```python
from build123d import *

# Parameters (mm, degrees)
F0_W      = 90
F0_H      = 19.25
F0_W_2    = 85
F0_H_2    = 12
F1_DEPTH  = 45
F0_W_3    = 7.85
F0_H_3    = 4.66
F2_DEPTH  = 14
F0_R      = 1.5
F3_DEPTH  = 8
F5_W      = 4
F5_H      = 29.0582341515
F6_DEPTH  = 3.07077
F5_H_2    = 15.9417658485
F7_DEPTH  = 8.2825263962
F11_DEPTH = 23.33121
F12_DEPTH = 2.5
F14_W     = 3
F14_H     = 4.4074529409
F14_W_2   = 3.907799057
F14_H_2   = 3
F15_DEPTH = 3


with BuildPart() as f1:
    # F0 (on Front) → F1 (new body)
    with BuildSketch(Plane.XZ):
        with Locations((-17.1932545304, 37.9297346771)):
            Rectangle(F0_W, F0_H)
        with Locations((-17.2074458234, 37.7867133319)):
            Rectangle(F0_W_2, F0_H_2, mode=Mode.SUBTRACT)
    extrude(amount=F1_DEPTH)

    # F0 (on Front) → F2 (join)
    with BuildSketch(Plane.XZ):
        with Locations((-17.2074458234, 37.7867133319)):
            Rectangle(F0_W_2, F0_H_2)
        with Locations((-17.2074458234, 37.7867133319)):
            Rectangle(F0_W_3, F0_H_3, mode=Mode.SUBTRACT)
    extrude(amount=F2_DEPTH)

    # F0 (on Front) → F3 (join)
    with BuildSketch(Plane.XZ):
        with Locations((-17.2074458234, 37.7867133319)):
            Rectangle(F0_W_3, F0_H_3)
        with Locations((-17.2074458234, 37.7867133319)):
            Circle(F0_R, mode=Mode.SUBTRACT)
    extrude(amount=F3_DEPTH)

    # F5 (on offset) → F6 (cut)
    with BuildSketch(Plane(origin=(0, 0, 28.3047346771), x_dir=(1, 0, 0), z_dir=(0, 0, -1))):
        with Locations((-17.1932545304, 30.4708829243)):
            Rectangle(F5_W, F5_H)
    extrude(amount=-F6_DEPTH, mode=Mode.SUBTRACT)

    # F5 (on offset) → F7 (cut)
    with BuildSketch(Plane(origin=(0, 0, 28.3047346771), x_dir=(1, 0, 0), z_dir=(0, 0, -1))):
        with Locations((-17.1932545304, 30.4708829243)):
            Rectangle(F5_W, F5_H)
        with Locations((-17.1932545304, 7.9708829243)):
            Rectangle(F5_W, F5_H_2)
    extrude(amount=-F7_DEPTH, mode=Mode.SUBTRACT)

    # F10 (on offset) → F11 (cut)
    with BuildSketch(Plane(origin=(0, 0, 28.3047346771), x_dir=(1, 0, 0), z_dir=(0, 0, -1))):
        with BuildLine():
            Line((-49.1650958551, 7.0774606429), (-45.4150958551, 7.0774606429))
            ThreePointArc((-45.4150958551, 7.0774606429), (-47.2900958551, 8.9524606429), (-49.1650958551, 7.0774606429))
        make_face()
        with BuildLine():
            ThreePointArc((-49.1650958551, 7.0774606429), (-47.2900958551, 5.2024606429), (-45.4150958551, 7.0774606429))
            Line((-45.4150958551, 7.0774606429), (-49.1650958551, 7.0774606429))
        make_face()
        with BuildLine():
            ThreePointArc((10.8743589147, 7.0774606429), (8.9993589147, 8.9524606429), (7.1243589147, 7.0774606429))
            Line((7.1243589147, 7.0774606429), (10.8743589147, 7.0774606429))
        make_face()
        with BuildLine():
            Line((10.8743589147, 7.0774606429), (7.1243589147, 7.0774606429))
            ThreePointArc((7.1243589147, 7.0774606429), (8.9993589147, 5.2024606429), (10.8743589147, 7.0774606429))
        make_face()
    extrude(amount=-F11_DEPTH, mode=Mode.SUBTRACT)

    # F10 (on offset) → F12 (cut)
    with BuildSketch(Plane(origin=(0, 0, 28.3047346771), x_dir=(1, 0, 0), z_dir=(0, 0, -1))):
        with BuildLine():
            Line((7.1243589147, 7.0774606429), (5.4493589147, 7.0774606429))
            ThreePointArc((5.4493589147, 7.0774606429), (8.9993589147, 3.5274606429), (12.5493589147, 7.0774606429))
            Line((12.5493589147, 7.0774606429), (10.8743589147, 7.0774606429))
            ThreePointArc((10.8743589147, 7.0774606429), (8.9993589147, 5.2024606429), (7.1243589147, 7.0774606429))
        make_face()
        with BuildLine():
            ThreePointArc((12.5493589147, 7.0774606429), (8.9993589147, 10.6274606429), (5.4493589147, 7.0774606429))
            Line((5.4493589147, 7.0774606429), (7.1243589147, 7.0774606429))
            ThreePointArc((7.1243589147, 7.0774606429), (8.9993589147, 8.9524606429), (10.8743589147, 7.0774606429))
            Line((10.8743589147, 7.0774606429), (12.5493589147, 7.0774606429))
        make_face()
        with BuildLine():
            Line((-43.7400958551, 7.0774606429), (-45.4150958551, 7.0774606429))
            ThreePointArc((-45.4150958551, 7.0774606429), (-47.2900958551, 5.2024606429), (-49.1650958551, 7.0774606429))
            Line((-49.1650958551, 7.0774606429), (-50.8400958551, 7.0774606429))
            ThreePointArc((-50.8400958551, 7.0774606429), (-47.2900958551, 3.5274606429), (-43.7400958551, 7.0774606429))
        make_face()
        with BuildLine():
            ThreePointArc((-49.1650958551, 7.0774606429), (-47.2900958551, 8.9524606429), (-45.4150958551, 7.0774606429))
            Line((-45.4150958551, 7.0774606429), (-43.7400958551, 7.0774606429))
            ThreePointArc((-43.7400958551, 7.0774606429), (-47.2900958551, 10.6274606429), (-50.8400958551, 7.0774606429))
            Line((-50.8400958551, 7.0774606429), (-49.1650958551, 7.0774606429))
        make_face()
    extrude(amount=-F12_DEPTH, mode=Mode.SUBTRACT)

    # F14 (on face) → F15 (cut)
    with BuildSketch(Plane.XZ):
        Polygon((-21.1324458234, 36.2700645477), (-21.1324458234, 39.2700645477), (-39.4217026339, 39.2700645477), (-39.4217026339, 43.7867133319), (-42.4217026339, 43.7867133319), (-42.4217026339, 39.2700645477), (-42.4217026339, 36.2700645477), (-39.4217026339, 36.2700645477), align=None)
        with Locations((-40.9217026339, 45.9904398024)):
            Rectangle(F14_W, F14_H)
        with Locations((-19.1785462949, 37.7700645477)):
            Rectangle(F14_W_2, F14_H_2)
    extrude(amount=F15_DEPTH, mode=Mode.SUBTRACT)


solid = f1.part
```
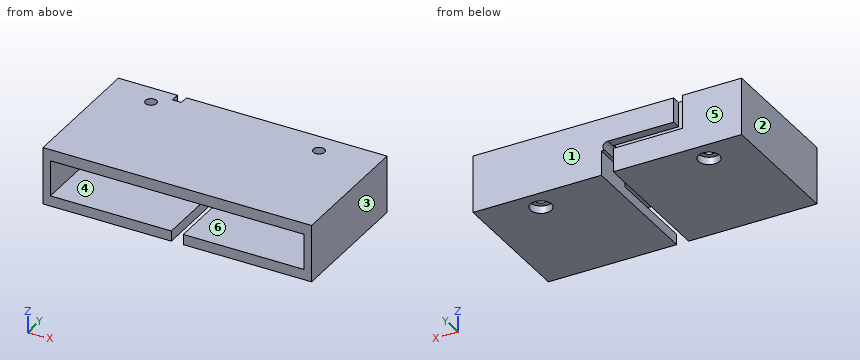
Source: CAD feature listing. Evaluate the final solid. Frame: model axes, mm. Face numbers are marked on the shaded views. A direction names the side the tool comes from. Give positions to 0.01 mm unless a question says otherwise; leave off trailing zeros. Loops run counter-clockwise (first coordinate to the right, second up) from the corner with the lowest first, then second, coordinate; pieces in that order, holes last. Notation, with made-up numbers: (71.5, -29) - (127.5, -29) arc R15 ccw to (127.5, -24) - close; hole circle Ø9 at (-5.75, 6.25). An arc over 180 degrees is marked (long way). Use CSV: the item, a comma, the result in double quotes.
1) Cut plane C-C (y = -11.5). Output: boundary loops of the cut face in (x, z), and give its area (3 significant figures).
Worked out:
outline,"(-62.19, 28.3) - (-19.19, 28.3) - (-19.19, 35.46) - (-21.13, 35.46) - (-21.13, 40.12) - (-13.28, 40.12) - (-13.28, 35.46) - (-15.19, 35.46) - (-15.19, 28.3) - (27.81, 28.3) - (27.81, 47.55) - (-62.19, 47.55) - close"
area,"1,670 mm^2"
2) Cut plane B-B (x = 18.5). Output: boundary loops of the cut face in (y, z), and give its area (3 significant figures).
Worked out:
outline,"(-45, 28.3) - (0, 28.3) - (0, 47.55) - (-45, 47.55) - (-45, 43.79) - (-14, 43.79) - (-14, 31.79) - (-45, 31.79) - close"
area,"494 mm^2"
3) Set-up query: the marked faces 5 and 6. Return all of +Z, -Z, +X, -X, +Y, -Y with unobstructed straight access to the full face (end or side cutting, diameter ignored); none if empty.
Worked out:
face 5,"+Z, -Z, +X, -X, +Y"
face 6,"-Y"
4) Mould query, pull axis X, two halves, no side actions, for the marked faces 1, 2, 3 and 4. Classes: +X half, -X half, draft (parallel to the pull), parting line (faces both ways), or undercut.
Worked out:
face 1,"draft"
face 2,"-X half"
face 3,"+X half"
face 4,"undercut"
5) Cut plane D-D (y = -19). Output: boundary loops of the cut face in (x, z).
Worked out:
outline,"(-62.19, 28.3) - (-19.19, 28.3) - (-19.19, 31.79) - (-59.71, 31.79) - (-59.71, 43.79) - (25.29, 43.79) - (25.29, 31.79) - (-15.19, 31.79) - (-15.19, 28.3) - (27.81, 28.3) - (27.81, 47.55) - (-62.19, 47.55) - close"
6) Line query: line 1 (Z direction, x = -35, y = -22.5); line 2 (X direction, y = -19.5, z = 41.25); line 3 (X direction, y = -5.5, z = 45.25). Output: solid intervals per line, ascending.
Worked out:
line 1,"z = 28.3 to 31.79, 43.79 to 47.55"
line 2,"x = -62.19 to -59.71, 25.29 to 27.81"
line 3,"x = -62.19 to -48.3, -46.28 to 7.99, 10.01 to 27.81"
7) Pin query (flat end, axial travel): P1, Ø6, axis at x = -47.29, y = -7.08, coming from the -Z side; P2, Ø3, axis at x = 9, y = -7.08, coming from the -Z side; P3, Ø5, axis at x = -15.5, z = 38.5, coming from the -Y side. Return the tip coordinate at first contact, or that it passes through.
Worked out:
P1,"stops at z = 30.8"
P2,"passes through"
P3,"stops at y = -14"
8) Cut plane A-A (x = 9). Output: boundary loops of the cut face in (y, z), and give its area (3 significant figures).
Worked out:
outline,"(-45, 28.3) - (-10.63, 28.3) - (-10.63, 30.8) - (-8.95, 30.8) - (-8.95, 47.55) - (-45, 47.55) - (-45, 43.79) - (-14, 43.79) - (-14, 31.79) - (-45, 31.79) - close; (-5.2, 30.8) - (-3.53, 30.8) - (-3.53, 28.3) - (0, 28.3) - (0, 47.55) - (-5.2, 47.55) - close"
area,"414 mm^2"
